Verification items for this drawing (mm, ordinates from the low corner). A direction names the side the tool comes from. Round coordinates to 2 decimals unless told otherwise and drop trailing zeros. Order: outer loops, then holes, each group sorted by start corner. A loop starts at its lowest first (then second) coordinate and runs counter-clockwise, first axis right, second up. Notation, with made-up numbers: (-4, 79) -> (14, 79) arc R7 ccw to (14, 85) -> close; hole circle Ø4 at (74.25, 35). An arc over 180 degrees is marked (long way). Answer in a Markdown table with one row per item. Add a question column.
1. Material ranges on L1, parallel to Z at x = 3.5, y = 25; L2, parallel to Y at x = 9, z = 99; L3, parallel to Z at x = 2.25, y = 20.5, recorded low to high. Write a range as from..to.
2. Access from +Z, -Z, +X, -X, +Y, -Y to the whole of each face (thin tool, end or side, straight path). Record for the marked faces 1 and 2.
3. Sectioned sample at C-C, the plane z = 71.5. Record the boundary of the cut face in (x, y), then the cut area to 3 significant figures.
4. Sectioned sample at B-B, the plane x = 2.25. Record the boundary of the cut face in (y, z).
5. Sectioned sample at A-A, the plane y = 31. Record the boundary of the cut face in (x, z).
6. Depth check by flat-ended pin: P1, Ø1.5, axis at x = 5.5, z = 56, coming from the -Y side. Enter the tip coordinate at first touch or a pass-through.
7. Draft check along Y on the marked faces 3, 4 and 5. Enter one of: +Y half, -Y half, draft (parallel to the pull), parting line (faces both ways), or undercut.
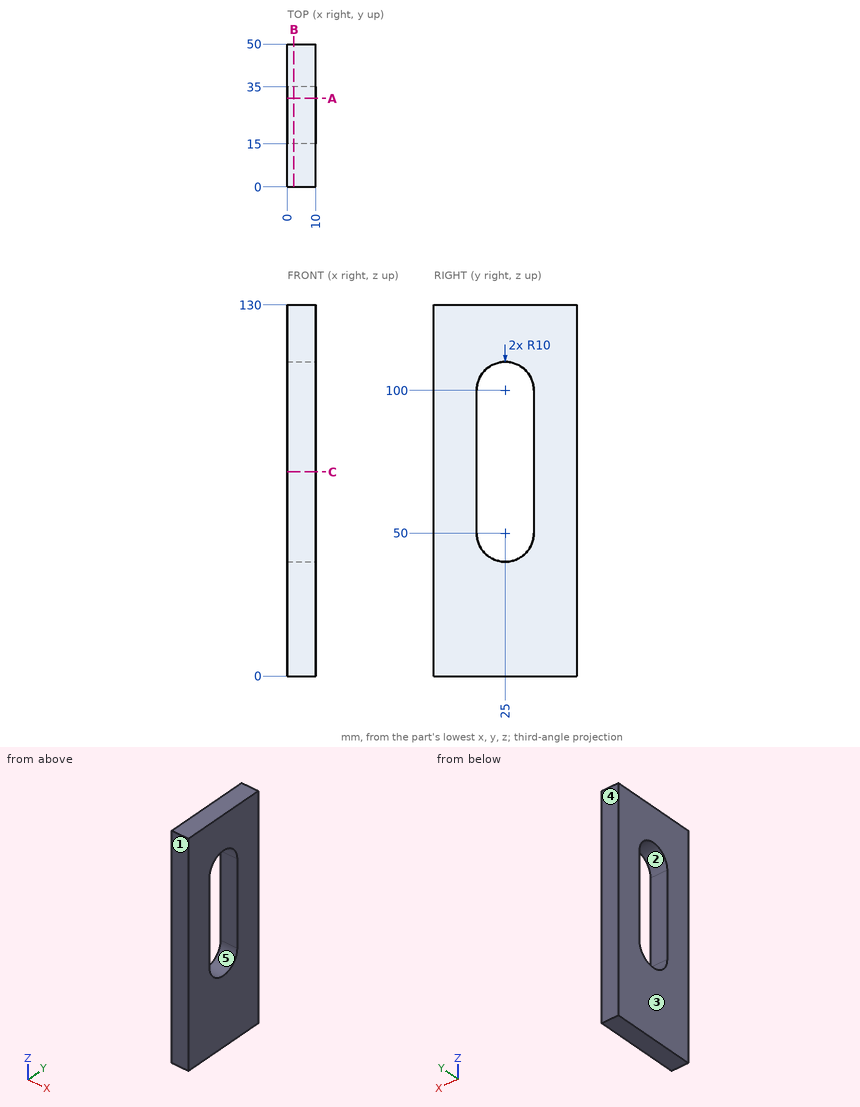
Answer key:
| question | item | result |
|---|---|---|
| 1 | L1 | z = 0..40, 110..130 |
| 1 | L2 | y = 0..15, 35..50 |
| 1 | L3 | z = 0..41.07, 108.93..130 |
| 2 | face 1 | +Z, -Z, +X, -X, -Y |
| 2 | face 2 | +X, -X |
| 3 | outline | (0, 0) -> (10, 0) -> (10, 15) -> (0, 15) -> close; (0, 35) -> (10, 35) -> (10, 50) -> (0, 50) -> close |
| 3 | area | 300 mm² |
| 4 | outline | (0, 0) -> (50, 0) -> (50, 130) -> (0, 130) -> close; hole (15, 50) arc R10 ccw to (35, 50) -> (35, 100) arc R10 ccw to (15, 100) -> close |
| 5 | outline | (0, 0) -> (10, 0) -> (10, 42) -> (0, 42) -> close; (0, 108) -> (10, 108) -> (10, 130) -> (0, 130) -> close |
| 6 | P1 | stops at y = 0 |
| 7 | face 3 | draft |
| 7 | face 4 | +Y half |
| 7 | face 5 | undercut |
